```python
from build123d import *

# Parameters (mm, degrees)
RESSALTO_EXTRUS_O1_DEPTH     = 3
FURO_DE_DI_METRO_3_0_3_1_D   = 3
FURO_DE_DI_METRO_2_6_2_6_1_D = 2.6


with BuildPart() as part:
    # Esboço1 → Ressalto-extrusão1 (new body)
    with BuildSketch(Plane(origin=(0, 0, 0), x_dir=(1, 0, 0), z_dir=(0, 1, 0))):
        with BuildLine():
            Line((-9, -4), (9, -4))
            ThreePointArc((9, -4), (13, 0), (9, 4))
            ThreePointArc((9, 4), (0.835034191, 5.742581416), (-5.90711985, 10.666666667))
            ThreePointArc((-5.90711985, 10.666666667), (-7.255550658, 11.651483717), (-8.88854382, 12))
            Line((-8.88854382, 12), (-9, 12))
            ThreePointArc((-9, 12), (-11.828427125, 10.828427125), (-13, 8))
            Line((-13, 8), (-13, 0))
            ThreePointArc((-13, 0), (-11.828427125, -2.828427125), (-9, -4))
        make_face()
    extrude(amount=RESSALTO_EXTRUS_O1_DEPTH)

    # Furo de diâmetro Ø3.0 (3)1 (through all)
    with Locations(Plane(origin=(0, 3, 0), x_dir=(1, 0, 0), z_dir=(0, 1, 0))):
        with Locations((9, 0)):
            Hole(FURO_DE_DI_METRO_3_0_3_1_D / 2)

    # Furo de diâmetro Ø2.6 (2.6)1 (through all)
    with Locations(Plane(origin=(0, 3, 0), x_dir=(1, 0, 0), z_dir=(0, 1, 0))):
        with Locations((-9, 0)):
            Hole(FURO_DE_DI_METRO_2_6_2_6_1_D / 2)


solid = part.part
```
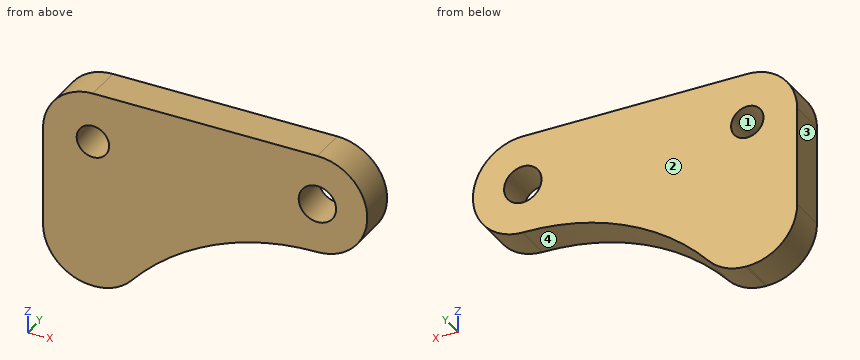
The listing builds one solid part. Answer for the finished solid, in the listing's coordinates (mm). Face numbers are marked on the shaded views. Give positions to 0.01 mm unless a question says otherwise; leave off trailing zeros. Order: outer loops, then holes, each group sorted by start corner. A loop starts at its lowest first (then second) coordinate and runs counter-clockwise, first axis right, second up. Notation, with made-up numbers: (77, -33.75) -> (83, -33.75) arc R20 ccw to (83, -10.75) -> close; hole circle Ø4 at (-22.75, 86.25). An arc over 180 degrees is marked (long way). Answer as a JSON object with one key per item and string values. Group by question number.
Item 1: The part is cut by section D-D on x = 11.75. Write down the section's boundary in (y, z), and give its area (3 significant figures).
Item 2: The part is cut by section A-A on y = 1.5. Write down the section's boundary in (x, z).
Item 3: The part is cut by section B-B on x = -8.5. Write down the section's boundary in (y, z).
Item 4: The part is cut by section C-C on z = -11. Write down the section's boundary in (x, y), and give its area (3 significant figures).
Item 5: Consider L1, parallel to Z at x = -9, y = 1.1; L2, parallel to Z at x = 9, y = 0.85; L3, parallel to Z at x = -3, y = 0.2. Determine where each line is inside the solid, lowest interval first. Write a range as from..to.
Item 6: A flat-ended cylindrical pin translates along its axis: pin 1 (1 mm diameter, centred on y = 2, z = -9, fed in from -X). Find the tip coordinate at first contact, or state that the pin passes through.
Item 7: Determine the mould class of the marked faces 1, 2, 3 and 4 for opening direction X: pulls with the +X half, pulls with the -X half, needs draft (parallel to the pull), parting line crosses it, or undercut.
Result set:
{
 "1": {"outline": "(0, -2.9) -> (3, -2.9) -> (3, 2.9) -> (0, 2.9) -> close", "area": "17.4 mm²"},
 "2": {"outline": "(-13, -8) arc R4 ccw to (-9, -12) -> (-8.89, -12) arc R4 ccw to (-5.91, -10.67) arc R20 cw to (9, -4) arc R4 ccw to (9, 4) -> (-9, 4) arc R4 ccw to (-13, 0) -> close; hole circle Ø2.6 at (-9, 0); hole circle Ø3 at (9, 0)"},
 "3": {"outline": "(0, -11.98) -> (3, -11.98) -> (3, -1.2) -> (0, -1.2) -> close; (0, 1.2) -> (3, 1.2) -> (3, 4) -> (0, 4) -> close"},
 "4": {"outline": "(-11.65, 0) -> (-6.24, 0) -> (-6.24, 3) -> (-11.65, 3) -> close", "area": "16.2 mm²"},
 "5": {"L1": "-12..-1.3, 1.3..4", "L2": "-4..-1.5, 1.5..4", "L3": "-8..4"},
 "6": {"pin 1": "x = -12.97"},
 "7": {"face 1": "undercut", "face 2": "needs draft", "face 3": "pulls with the -X half", "face 4": "pulls with the +X half"}
}
